from build123d import *

# Parameters (mm, degrees)
SKETCH_1_R          = 21.9
SKETCH_1_R_2        = 20
EXTRUDE_1_DEPTH     = 20
EXTRUDE_2_DEPTH     = 33
SKETCH_8_OUTSIDE_W  = 120.99
SKETCH_8_OUTSIDE_H  = 110.78
SKETCH_8_OUTSIDE_R  = 33
CUT_EXTRUDE_4_DEPTH = 10
CUT_EXTRUDE_4_DRAFT = -45
SKETCH_9_OUTSIDE_W  = 120.99
SKETCH_9_OUTSIDE_H  = 110.78
SKETCH_9_OUTSIDE_R  = 33
CUT_EXTRUDE_5_DEPTH = 10
CUT_EXTRUDE_5_DRAFT = -45
SKETCH_10_R         = 29.7
CUT_EXTRUDE_6_DEPTH = 27.7
SKETCH_11_R         = 20
CUT_EXTRUDE_7_DEPTH = 58.517736395


with BuildPart() as part:
    # Эскиз1 → Вытянуть-Тонкостенный1 (new body)
    with BuildSketch(Plane(origin=(0, 0, 0), x_dir=(0, 0, -1), z_dir=(1, 0, 0))):
        Circle(SKETCH_1_R)
        Circle(SKETCH_1_R_2, mode=Mode.SUBTRACT)
    extrude(amount=EXTRUDE_1_DEPTH)

    # Эскиз2 → Бобышка-Вытянуть2 (add)
    with BuildSketch(Plane(origin=(20, 0, 0), x_dir=(0, 0, -1), z_dir=(1, 0, 0))):
        Polygon((38.105117767, 0), (19.052558883, 33), (-19.052558883, 33), (-38.105117767, 0), (-19.052558883, -33), (19.052558883, -33), align=None)
    extrude(amount=EXTRUDE_2_DEPTH)


with BuildPart() as cut_extrude_4_tool:
    # Эскиз8 outside → Вырез-Вытянуть4 (with draft: the straight prism first)
    with BuildSketch(Plane.ZY.offset(-20)):
        Rectangle(SKETCH_8_OUTSIDE_W, SKETCH_8_OUTSIDE_H)
        Circle(SKETCH_8_OUTSIDE_R, mode=Mode.SUBTRACT)
    extrude(amount=-CUT_EXTRUDE_4_DEPTH)
    # Вырез-Вытянуть4: the draft: its side faces are tilted about the plane it starts from
    cut_extrude_4_sides = [cut_extrude_4_tool.faces().sort_by_distance(p)[0] for p in [
        (25, -55.39, 0),
        (25, 0, 60.495),
        (25, 55.39, 0),
        (25, 0, -60.495),
        (25, 0, -33),
    ]]
    draft(cut_extrude_4_sides, Plane.ZY.offset(-20), CUT_EXTRUDE_4_DRAFT)


with BuildPart() as part_1:
    add(part.part)

    # Вырез-Вытянуть4: cut by cut_extrude_4_tool
    add(cut_extrude_4_tool.part, mode=Mode.SUBTRACT)


with BuildPart() as cut_extrude_5_tool:
    # Эскиз9 outside → Вырез-Вытянуть5 (with draft: the straight prism first)
    with BuildSketch(Plane(origin=(53, 0, 0), x_dir=(0, 0, -1), z_dir=(1, 0, 0))):
        Rectangle(SKETCH_9_OUTSIDE_W, SKETCH_9_OUTSIDE_H)
        Circle(SKETCH_9_OUTSIDE_R, mode=Mode.SUBTRACT)
    extrude(amount=-CUT_EXTRUDE_5_DEPTH)
    # Вырез-Вытянуть5: the draft: its side faces are tilted about the plane it starts from
    cut_extrude_5_sides = [cut_extrude_5_tool.faces().sort_by_distance(p)[0] for p in [
        (48, -55.39, 0),
        (48, 0, -60.495),
        (48, 55.39, 0),
        (48, 0, 60.495),
        (48, 0, 33),
    ]]
    draft(cut_extrude_5_sides, Plane(origin=(53, 0, 0), x_dir=(0, 0, -1), z_dir=(1, 0, 0)), CUT_EXTRUDE_5_DRAFT)


with BuildPart() as part_2:
    add(part_1.part)

    # Вырез-Вытянуть5: cut by cut_extrude_5_tool
    add(cut_extrude_5_tool.part, mode=Mode.SUBTRACT)

    # Эскиз10 → Вырез-Вытянуть6 (cut)
    with BuildSketch(Plane(origin=(53, 0, 0), x_dir=(0, 0, -1), z_dir=(1, 0, 0))):
        Circle(SKETCH_10_R)
    extrude(amount=-CUT_EXTRUDE_6_DEPTH, mode=Mode.SUBTRACT)

    # Эскиз11 → Вырез-Вытянуть7 (cut, through all)
    with BuildSketch(Plane(origin=(25.3, 0, 0), x_dir=(0, 0, -1), z_dir=(1, 0, 0))):
        Circle(SKETCH_11_R)
    extrude(amount=-CUT_EXTRUDE_7_DEPTH, mode=Mode.SUBTRACT)


solid = part_2.part
Geometry: final body of the model. Coordinates: model frame, mm. A direction names the side the tool comes from. Give positions to 0.01 mm unless a question says otherwise; leave off trailing zeros. Write each loop counter-clockwise with the first axis right and the second up, starting at its lowest first coordinate (ties: lowest second). Pieces come first, ordered by that corner, then holes. Notation, with made-up numbers: (19.5, -30) -> (67.5, -30) arc R10 ccw to (67.5, -23) -> close; hole circle Ø2 at (-25.5, 41). An arc over 180 degrees is marked (long way). Answer in a Markdown table with one row per item.
(1) Pin query (flat end, axial travel): pin 1 (1 mm diameter, centred on y = -21, z = 21.5, fed in from -X); pin 2 (10 mm diameter, centred on x = 34.5, y = -6, fed in from -Z); pin 3 (6 mm diameter, centred on x = 47.5, y = 26.5, fed in from +Z). Return the tip coordinate at first contact, or that it passes through.
Answers below:
| item | result |
|---|---|
| pin 1 | x = 20 |
| pin 2 | z = -37.53 |
| pin 3 | z = 24.54 |
(2) Ray query, line 1 along Y through (x, z) = (41.25, 0); line 2 along Z through (x, y) = (42, 9); line 3 along Y through (x, z) = (37.5, -22.5). Return the intervals inside material, ascending. Write a range as [from, to].
Answers below:
| item | result |
|---|---|
| line 1 | [-33, -29.7], [29.7, 33] |
| line 2 | [-32.91, -28.3], [28.3, 32.91] |
| line 3 | [-27.03, -19.39], [19.39, 27.03] |
(3) Section query A-A on x = 13. Return loops of the section in (y, z).
Answers below:
| item | result |
|---|---|
| outline | circle Ø43.8 at (0, 0); hole circle Ø40 at (0, 0) |
(4) Set-up query: faces 1 (the flat face through (20, -7, -22)), 2 (the flat face through (36.27, -16.27, 28.71)). Return all of +Z, -Z, +X, -X, +Y, -Y with unobstructed straight access to the full face (end or side cutting, diameter ignored); none if empty.
Answers below:
| item | result |
|---|---|
| face 1 | -X |
| face 2 | +Z, +X, -X, -Y |
(5) Draft query along Y for faces 3 (the cylindrical face through (12.473, -19.524, 4.336)), 4 (the flat face through (25.3, -19.4, -6.2)), 5 (the conical face through (51.783, -29.591, 17.181)), 6 (the conical face through (21.217, 29.675, -17.036)). Return one class per face: +Y half, -Y half, draft (parallel to the pull), parting line (faces both ways), or undercut.
Answers below:
| item | result |
|---|---|
| face 3 | undercut |
| face 4 | undercut |
| face 5 | -Y half |
| face 6 | +Y half |
(6) Section query B-B on x = 21. Return loops of the section in (y, z), then the cut area to 3 significant figures.
Answers below:
| item | result |
|---|---|
| outline | (-33, -8.19) arc R34 ccw to (-23.59, -24.49) -> (-9.41, -32.67) arc R34 ccw to (9.41, -32.67) -> (23.59, -24.49) arc R34 ccw to (33, -8.19) -> (33, 8.19) arc R34 ccw to (23.59, 24.49) -> (9.41, 32.67) arc R34 ccw to (-9.41, 32.67) -> (-23.59, 24.49) arc R34 ccw to (-33, 8.19) -> close; hole circle Ø40 at (0, 0) |
| area | 2,310 mm^2 |
